The listing builds one solid part. Answer for the finished solid, in the listing's coordinates (mm). A direction names the side the tool comes from. Coordinates: 2 decimals unless noted, no trailing zeros. Loops run counter-clockwise (first coordinate to the right, second up) from the corner with the lowest first, then second, coordinate; pieces in that order, holes last. Notation, with made-up numbers: M 31,23.25 L 35,23.25 A28 ccw 35,44.25 Z; hole C 51,82 d6. An arc over 180 degrees is marked long. Return JSON: item names as keys, results as strings. Group by question number.
1. Section B-B (y = -2.35) is taken. Write down the section's boundary in (x, z).
2. The mould has two halves that part along Z. Classify faces 3 (the face through (-5.1, 1.5, 5.4)), 4 (the face through (0, 0, 0)), 5 (the face through (0, 0, 8)): pulls with the +Z half, pulls with the -Z half, needs draft (parallel to the pull), parting line crosses it, or undercut.
3. Section A-A (y = -0.5) is taken. Write down the section's boundary in (x, z).
4. Straight lines are drawn through the part: L1, parallel to Z at x = 4, y = -0.3; L2, parallel to Y at x = 4, z = 6.5. For each, find the intervals that lie inside material, in ascending order. Write a range as from..to.
5. Which of the six approach directions +Z, -Z, +X, -X, +Y, -Y give full straight-line access (tool end or side, diameter ignored) to faces 1 (the face through (7.644, -0.014, 7.624)), 2 (the face through (3, -1, -1.48))?
6. Given P1, Ø1.5, axis at y = -1.5, z = -0.5, coming from the -X side; P2, Ø1.5, axis at x = -4, z = 5.5, coming from the -Y side, each flat-ended and moving along its own axis, determine where each tip first touches the part or whether it passes through.
Autodesk Fusion 360 part; units mm, degrees
sketch "plan" plane through (0, 0, 0) normal (0, 1, 0) x (1, 0, 0)
  line L0 (8, 8) -> (-8, 8)
  line L1 (-8, 8) -> (-8, -8)
  line L2 (-8, -8) -> (8, -8)
  line L3 (8, -8) -> (8, 8)
  line L4 (7, 7) -> (-7, 7)
  line L5 (-7, 7) -> (-7, -7)
  line L6 (-7, -7) -> (7, -7)
  line L7 (7, -7) -> (7, 7)
  line L8 (-3.48, 0) -> (3.48, 0) construction
  line L9 (-3.48, -1.48) -> (-2.2, -1.48)
  line L10 (-2.2, -1.48) -> (-2.2, 1.48)
  line L11 (-2.2, 1.48) -> (-3.48, 1.48)
  line L12 (-3.48, 1.48) -> (-3.48, -1.48)
  line L13 (-7, 7) -> (7, -7) construction
  line L14 (-8, -8) -> (8, 8) construction
  line L15 (2.2, -1.48) -> (3.48, -1.48)
  line L16 (3.48, -1.48) -> (3.48, 1.48)
  line L17 (3.48, 1.48) -> (2.2, 1.48)
  line L18 (2.2, 1.48) -> (2.2, -1.48)
  dimension "d1" = 16
  dimension "d2" = 16
  dimension "d3" = 1
  dimension "d5" = 1
  dimension "d10" = 6.96
  dimension "d11" = 1.28
  dimension "d12" = 2.96
  dimension "d13" = 1.28
  dimension "d14" = 2.96
extrude "Extrude1" add sketch "plan" along normal blind 1.5 contours L0 L1 L2 L3 | L4 L5 L6 L7 | L9 L10 L11 L12 | L15 L16 L17 L18
extrude "Extrude2" add sketch "plan" against normal blind 1 contours L0 L1 L2 L3
extrude "Extrude3" add sketch "plan" against normal blind 2.96 contours L9 L10 L11 L12 | L15 L16 L17 L18
sketch "indent" plane through (0, 0, 0) normal (0, 0, 1) x (1, 0, 0)
  line L0 (8, -1) -> (8, 1.5)
  line L1 (8, 1.5) -> (8, -1)
  line L2 (8, 1.5) -> (-8, 1.5)
  line L3 (-8, 1.5) -> (8, 1.5)
  line L4 (-8, -1) -> (-8, 1.5)
  line L5 (-8, 1.5) -> (-8, -1)
  line L6 (-8, 0) -> (8, 0)
  line L7 (0, 1.5) -> (0, 0.7)
  spline S0 degree 5 poles (-6.4, 1.5) (-6.144, 1.4393) (-5.632, 1.3233) (-4.864, 1.1651) (-3.84, 0.9865) (-2.56, 0.8208) (-1.28, 0.7177) (0, 0.6824) (1.28, 0.7177) (2.56, 0.8208) (3.84, 0.9865) (4.864, 1.1651) (5.632, 1.3233) (6.144, 1.4393) (6.4, 1.5) knots 0 0 0 0 0 0 0.1 0.2 0.3 0.4 0.5 0.6 0.7 0.8 0.9 1 1 1 1 1 1
  point P0 (-8, 0)
  point P1 (8, 0)
  point P2 (-6.4, 1.5)
  point P3 (6.4, 1.5)
  dimension "d17" = 1.6
  dimension "d18" = 1.6
  dimension "d20" = 0.8
revolve "Revolve1" cut sketch "indent" angle 360 about axis through (0, 1.75, 0) along (0, 1, 0) contours L2 L3 L7 S0 picked at (0.7111, 0.9984)
fillet "Fillet1" radius 1.25 4 edges at (-8, 0.25, 8) (8, 0.25, 8) (8, 0.25, -8) (-8, 0.25, -8)
fillet "Fillet2" radius 0.5 8 edges at (7.6339, 1.5, -7.6339) (0, 1.5, -8) (-7.6339, 1.5, -7.6339) (-8, 1.5, 0) (-7.6339, 1.5, 7.6339) (0, 1.5, 8) (7.6339, 1.5, 7.6339) (8, 1.5, 0)
fillet "Fillet3" radius 7 1 edges at (-5.9669, 1.5, -2.3143)
equation "d13 = d11"
equation "d14 = d12"
equation "d18 = d17"
Worked out:
{
 "1": {"outline": "M -3.48,-1.48 L -2.2,-1.48 L -2.2,1.48 L -3.48,1.48 Z; M 2.2,-1.48 L 3.48,-1.48 L 3.48,1.48 L 2.2,1.48 Z"},
 "2": {"face 3": "needs draft", "face 4": "undercut", "face 5": "pulls with the +Z half"},
 "3": {"outline": "M -8,-6.75 A1.25 ccw -6.75,-8 L 6.75,-8 A1.25 ccw 8,-6.75 L 8,6.75 A1.25 ccw 6.75,8 L -6.75,8 A1.25 ccw -8,6.75 Z; M -3.48,-1.48 L -2.2,-1.48 L -2.2,1.48 L -3.48,1.48 Z; M 2.2,-1.48 L 3.48,-1.48 L 3.48,1.48 L 2.2,1.48 Z; hole M -7,-7 L 7,-7 L 7,7 L -7,7 Z"},
 "4": {"L1": "-8..-7, 7..8", "L2": "0..1.5"},
 "5": {"face 1": "+Z, +X, +Y, -Y", "face 2": "-Y"},
 "6": {"P1": "x = -8", "P2": "y = 0"}
}
